```python
from build123d import *

# Parameters (mm, degrees)
BASES_R            = 21
BASES_R_2          = 17
BASE_DEPTH         = 4
FLATCUT_DEPTH      = 30.966648128
FCCIRPATTERN_COUNT = 4
BASECHAMFER_SIZE   = 0.2


with BuildPart() as part:
    # BaseS → Base (new, symmetric)
    with BuildSketch(Plane(origin=(0, 0, 0), x_dir=(1, 0, 0), z_dir=(0, 1, 0))):
        with Locations(Location((0, 0, 0), (0, 0, 270))):
            Circle(BASES_R)
        with Locations(Location((0, 0, 0), (0, 0, 270))):
            Circle(BASES_R_2, mode=Mode.SUBTRACT)
    extrude(amount=BASE_DEPTH, both=True)

    # FlatCutS → FlatCut (cut, symmetric)
    with BuildSketch(Plane(origin=(0, 0, 0), x_dir=(1, 0, 0), z_dir=(0, 1, 0))):
        with BuildLine():
            Line((11.274664333, 17.716713696), (17.716713696, 11.274664333))
            ThreePointArc((17.716713696, 11.274664333), (14.849242405, 14.849242405), (11.274664333, 17.716713696))
        make_face()
    flatcut = extrude(amount=FLATCUT_DEPTH, both=True, mode=Mode.SUBTRACT)

    # FCCirPattern: FlatCut ×4 about axis
    fccirpattern_axis = Axis((0, 0, 0), (0, 1, 0))
    for i in range(1, FCCIRPATTERN_COUNT):
        add(flatcut.rotate(fccirpattern_axis, i * 360 / FCCIRPATTERN_COUNT), mode=Mode.SUBTRACT)

    # BaseChamfer
    basechamfer_edges = [part.edges().sort_by_distance(p)[0] for p in [
        (0, -4, -17),
        (0, 4, -17),
    ]]
    chamfer(basechamfer_edges, length=BASECHAMFER_SIZE)


solid = part.part
```
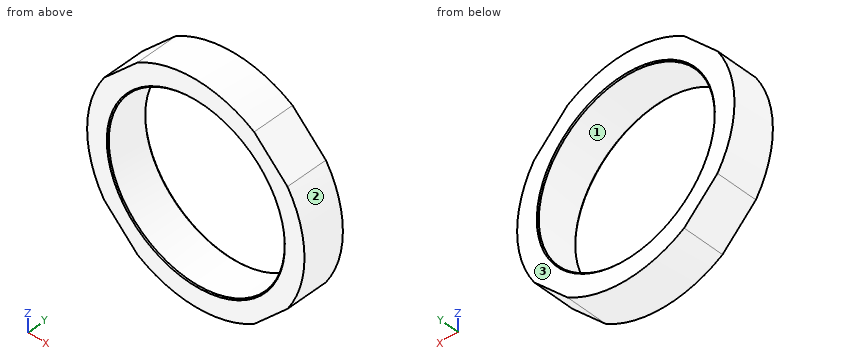
Design review of the part built by this model. Coordinates are the model's own, in mm. Face numbers are marked on the shaded views. Coordinates: 2 decimals unless noted, no trailing zeros. Write each loop counter-clockwise with the first axis right and the second up, starting at its lowest first coordinate (ties: lowest second). Pieces come first, ordered by that corner, then holes. Notation, with made-up numbers: M 16.25,8.25 L 24.25,8.25 A5 ccw 24.25,16.25 Z; hole C 18,53.5 d3. An arc over 180 degrees is marked long. Answer as a JSON object with one key per item and string values.
Item 1: Add section B-B, the plane z = 0. Give the boundary of the cut face in (x, y), and give its area (3 significant figures).
Outcome:
{"outline": "M -21,-4 L -17.2,-4 L -17,-3.8 L -17,3.8 L -17.2,4 L -21,4 Z; M 17,-3.8 L 17.2,-4 L 21,-4 L 21,4 L 17.2,4 L 17,3.8 Z", "area": "63.9 mm²"}
Item 2: Add section A-A, the plane x = 0. Give the boundary of the cut face in (y, z), and give its area (3 significant figures).
Outcome:
{"outline": "M -4,-21 L 4,-21 L 4,-17.2 L 3.8,-17 L -3.8,-17 L -4,-17.2 Z; M -4,17.2 L -3.8,17 L 3.8,17 L 4,17.2 L 4,21 L -4,21 Z", "area": "63.9 mm²"}
Item 3: Draft analysis for pull direction Z (two halves, no side actions). For the marked faces 1, 2 and 3, state which applies: pulls with the +Z half, pulls with the -Z half, needs draft (parallel to the pull), parting line crosses it, or undercut.
Outcome:
{"face 1": "undercut", "face 2": "parting line crosses it", "face 3": "needs draft"}
Item 4: Add section C-C, the plane y = 2.75. Give the boundary of the cut face in (x, z).
Outcome:
{"outline": "M -17.72,-11.27 L -11.27,-17.72 A21 ccw 11.27,-17.72 L 17.72,-11.27 A21 ccw 17.72,11.27 L 11.27,17.72 A21 ccw -11.27,17.72 L -17.72,11.27 A21 ccw Z; hole C 0,0 d34"}
Item 5: Insertion check: pin 1 Ø3 at (x, y) = (14.5, -1.5) entering from +Z; pin 2 Ø4 at (x, y) = (-14, 2) entering from -Z; pin 3 Ø1 at (y, z) = (-0.5, 14.5) entering from +X. Each pin has a flat end and moves straight along its axis. Give the tip position at first contact, or say it passes through.
Outcome:
{"pin 1": "z = 15.99", "pin 2": "z = -16.99", "pin 3": "x = 14.99"}
Item 6: Wall thickness on probe 1 along X at (y, z) = (-1, 0); probe 2 along Z at (x, y) = (-0.5, 3.25); probe 3 along Z at (x, y) = (15, -0.25): over which ranges is each line inside the solid? List them lowest first.
Outcome:
{"probe 1": "-21 to -17, 17 to 21", "probe 2": "-20.99 to -16.99, 16.99 to 20.99", "probe 3": "-13.99 to -8, 8 to 13.99"}
